Answer from the drawing. Dimensions are ordinates in mm from the lowest x, y and z of the part. A direction names the side the tool comes from. Coordinates: 2 decimals unless noted, no trailing zeros. Write each loop counter-clockwise with the first axis right and the second up, starting at its lowest first coordinate (ties: lowest second). Pieces come first, ordered by that corner, then holes.
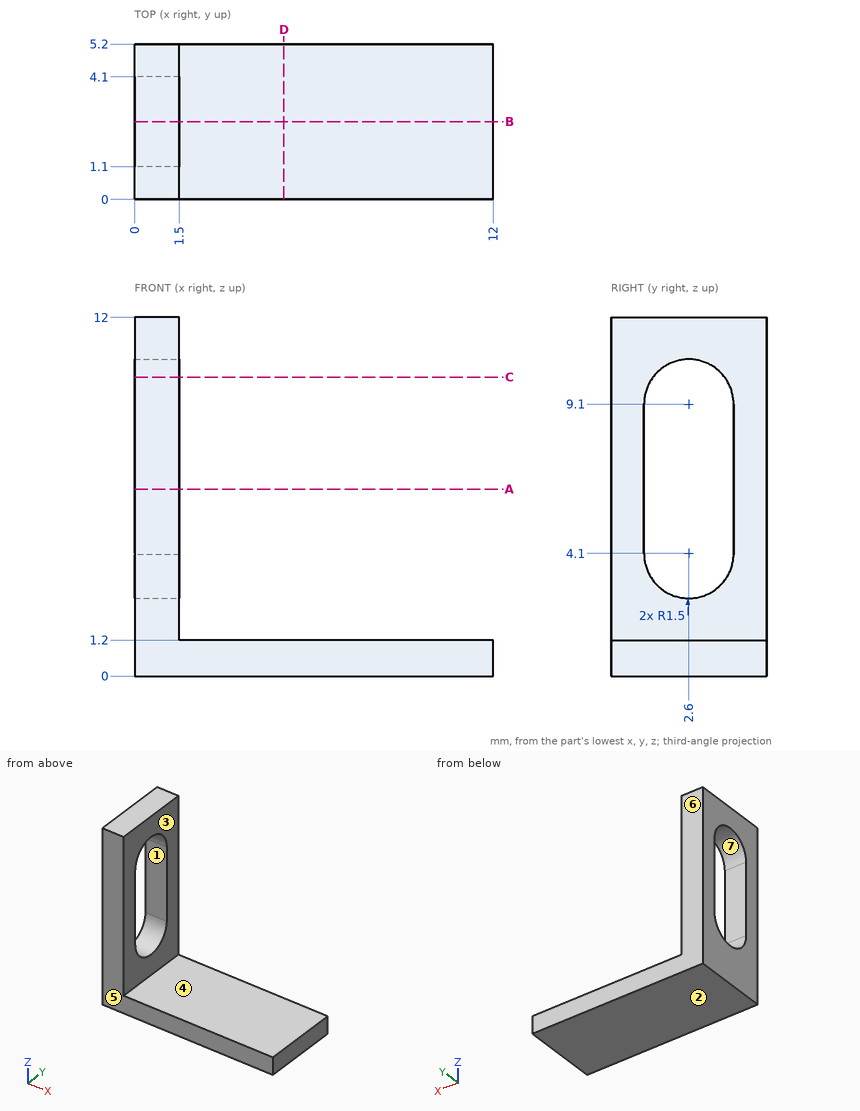
(1) Which of the six approach directions +Z, -Z, +X, -X, +Y, -Y give full straight-line access (tool end or side, diameter ignored) to the marked faces 1, 2 and 3?
(2) Section D-D, the plane x = 5 is taken. Write down the section's boundary in (y, z).
(3) Find the intervals of material crossed by probe 1 along Z at (x, y) = (0.75, 2.65); probe 2 along Z at (x, y) = (7, 2.15); probe 3 along X at (y, z) = (1.9, 1.25), in increasing order.
(4) For a pull along Y with two mould halves and no side action, classify the marked faces 4, 5, 6 and 7 as pulls with the +Y half, pulls with the -Y half, needs draft (parallel to the pull), parting line crosses it, or undercut.
(5) Each of these flat-tipped pins is pushed along its axis until it touches: pin 1 (1 mm diameter, centred on x = 8.5, y = 3, fed in from +Z); pin 2 (4 mm diameter, centred on x = 1.5, z = 5.5, fed in from -Y); pin 3 (2.5 mm diameter, centred on y = 3.5, z = 5, fed in from +X). Where does it stop, or does it pass through?
(6) Section C-C, the plane z = 10 is taken. Write down the section's boundary in (x, y).
(7) Section A-A, the plane z = 6.25 is taken. Write down the section's boundary in (x, y).
(8) Section B-B, the plane y = 2.6 is taken. Write down the section's boundary in (x, z), plus the area to 3 significant figures.
Solution:
1. face 1: +X, -X
1. face 2: -Z, +X, -X, +Y, -Y
1. face 3: +Z, +X, +Y, -Y
2. outline: (0, 0) - (5.2, 0) - (5.2, 1.2) - (0, 1.2) - close
3. probe 1: z = 0 to 2.6, 10.6 to 12
3. probe 2: z = 0 to 1.2
3. probe 3: x = 0 to 1.5
4. face 4: needs draft
4. face 5: pulls with the -Y half
4. face 6: pulls with the +Y half
4. face 7: undercut
5. pin 1: stops at z = 1.2
5. pin 2: stops at y = 0
5. pin 3: stops at x = 1.5
6. outline: (0, 0) - (1.5, 0) - (1.5, 1.4) - (0, 1.4) - close; (0, 3.8) - (1.5, 3.8) - (1.5, 5.2) - (0, 5.2) - close
7. outline: (0, 0) - (1.5, 0) - (1.5, 1.1) - (0, 1.1) - close; (0, 4.1) - (1.5, 4.1) - (1.5, 5.2) - (0, 5.2) - close
8. outline: (0, 0) - (12, 0) - (12, 1.2) - (1.5, 1.2) - (1.5, 2.6) - (0, 2.6) - close; (0, 10.6) - (1.5, 10.6) - (1.5, 12) - (0, 12) - close
8. area: 18.6 mm2
